from build123d import *

# Parameters (mm, degrees)
BOSS_EXTRUDE1_DEPTH     = 6.35
F_1_4_CLEARANCE_HOLE1_D = 6.7564
CUT_EXTRUDE1_DEPTH      = 7.35
FILLET1_R               = 1.5875
FILLET2_R               = 12.7
SKETCH7_R               = 3.175
CUT_EXTRUDE2_DEPTH      = 7.35


with BuildPart() as part:
    # Sketch3 → Boss-Extrude1 (new body)
    with BuildSketch(Plane.XY):
        Polygon((0, 0), (0, 72.39), (-134.112, 72.39), (-134.112, 0), (-115.062, 0), (-115.062, 46.99), (-69.85, 46.99), (-69.85, 0), align=None)
    extrude(amount=BOSS_EXTRUDE1_DEPTH)

    # 1/4 Clearance Hole1 (through all)
    with Locations(Plane.XY.offset(6.35)):
        with Locations((-50.8, 22.225), (-12.7, 22.225)):
            Hole(F_1_4_CLEARANCE_HOLE1_D / 2)

    # Sketch6 → Cut-Extrude1 (cut, through all)
    with BuildSketch(Plane.XY.offset(6.35)):
        Polygon((0, 72.39), (0, 40.64), (-38.1, 72.39), align=None)
    extrude(amount=-CUT_EXTRUDE1_DEPTH, mode=Mode.SUBTRACT)

    # Fillet1
    fillet1_edges = [part.edges().sort_by_distance(p)[0] for p in [
        (-69.85, 0, 3.175),
        (-115.062, 0, 3.175),
        (-134.112, 0, 3.175),
        (0, 0, 3.175),
    ]]
    fillet(fillet1_edges, radius=FILLET1_R)

    # Fillet2
    fillet2_edges = [part.edges().sort_by_distance(p)[0] for p in [
        (-134.112, 72.39, 3.175),
        (-38.1, 72.39, 3.175),
        (0, 40.64, 3.175),
    ]]
    fillet(fillet2_edges, radius=FILLET2_R)

    # Sketch7 → Cut-Extrude2 (cut, through all)
    with BuildSketch(Plane.XY.offset(6.35)):
        with Locations((-112.81693597, 44.74493597)):
            Circle(SKETCH7_R)
        with Locations((-72.09506403, 44.74493597)):
            Circle(SKETCH7_R)
    extrude(amount=-CUT_EXTRUDE2_DEPTH, mode=Mode.SUBTRACT)


solid = part.part
Geometry: final body of the model. Coordinates: model frame, mm. A direction names the side the tool comes from. Give positions to 0.01 mm unless a question says otherwise; leave off trailing zeros. Order: outer loops, then holes, each group sorted by start corner. A loop starts at its lowest first (then second) coordinate and runs counter-clockwise, first axis right, second up. Notation, with made-up numbers: (61, 33) -> (88, 33) arc R24 ccw to (88, 50) -> close; hole circle Ø3 at (-16.75, 30). An arc over 180 degrees is marked (long way). Put each result on its own line as item: value.
Q1. Section A-A, the plane x = -50.8. Return loops of the section in (y, z).
Here are the results:
outline: (0, 0) -> (18.85, 0) -> (18.85, 6.35) -> (0, 6.35) -> close; (25.6, 0) -> (72.39, 0) -> (72.39, 6.35) -> (25.6, 6.35) -> close
Q2. Section C-C, the plane z = 4. Count the separate pieces of the cut face and the enclosed holes in it, then the cut area to 3 significant figures.
Here are the results:
separate pieces: 1
enclosed holes: 2
area: 6,850 mm^2
Q3. Section D-D, the plane x = -99. Return loops of the section in (y, z), then the cut area to 3 significant figures.
Here are the results:
outline: (46.99, 0) -> (72.39, 0) -> (72.39, 6.35) -> (46.99, 6.35) -> close
area: 161 mm^2
Q4. Material intervals for L1, parallel to Y at x = -50.8, z = 3.25; L2, parallel to X at y = 33, z = 1.75; L3, parallel to X at y = 38.5, z = 4.75, sorted ascending.
Here are the results:
L1: y = 0 to 18.85, 25.6 to 72.39
L2: x = -134.11 to -115.06, -69.85 to 0
L3: x = -134.11 to -115.06, -69.85 to -0.58
Q5. Draft query along Y for faces 3 (the face through (-115.062, 22, 3)), 4 (the face through (-125, 0, 3)), 5 (the face through (-50.068, 18.927, 3.131)). Return one class per face: released by +Y, released by -Y, zero draft, split by the parting line, or undercut.
Here are the results:
face 3: zero draft
face 4: released by -Y
face 5: undercut
Q6. Reachability of faces 1 (the face through (-69.85, 22, 3)), 2 (the face through (-19.359, 56.772, 3.219)) from +Z, -Z, +X, -X, +Y, -Y: full face, straight path, thin tool, end or side. Return the list, or none.
Here are the results:
face 1: +Z, -Z, -Y
face 2: +Z, -Z, +X, +Y
Q7. Section B-B, the plane y = 31. Return loops of the section in (x, z).
Here are the results:
outline: (-134.11, 0) -> (-115.06, 0) -> (-115.06, 6.35) -> (-134.11, 6.35) -> close; (-69.85, 0) -> (0, 0) -> (0, 6.35) -> (-69.85, 6.35) -> close
Q8. Pin query (flat end, axial travel): pin 1 (1.9 mm diameter, centred on x = -95.5, z = 2, fed in from -Y). Return the tip coordinate at first contact, or that it passes through.
Here are the results:
pin 1: stops at y = 46.99
